Build history of the part. All positions in model axes, mm. Face numbers are marked on the shaded views. A direction names the side the tool comes from. Give positions to 0.01 mm unless a question says otherwise; leave off trailing zeros. Loops run counter-clockwise (first coordinate to the right, second up) from the corner with the lowest first, then second, coordinate; pieces in that order, holes last. Notation, with made-up numbers: (61.25, -15.75) -> (96.25, -15.75) arc R14 ccw to (96.25, -9.75) -> close; hole circle Ø10 at (57, 53.25). An arc over 180 degrees is marked (long way). Answer as a JSON object with one key per item and string values. Group by question number.
Q1. Band-saw the part on D-D, the plane x = 16.5. Write the cut outline in (y, z), plus the area to 3 significant figures.
Q2. Drop flat-ended pins along their axis: pin 1 (2 mm diameter, centred on x = -13, z = -2, fed in from +Y); pin 2 (2 mm diameter, centred on x = -8.5, y = 1, fed in from -Z); pin 3 (2 mm diameter, centred on y = 2.5, z = -8, fed in from -X); pin 4 (1.8 mm diameter, centred on y = 2.5, z = 5, fed in from -X). Give the stop position or say it passes through.
Q3. Wall check: probe 1 along X at (y, z) = (1.75, -5); probe 2 along X at (y, z) = (3.7, 5.5); probe 3 along Z at (x, y) = (13.5, 2.7). Give the ranges that are in metal, low to high. Write a range as from..to.
Q4. Band-saw the part on B-B, the plane y = 3. Write the cut outline in (x, z), plus the area to 3 significant figures.
Q5. Two-plate mould, pull along Z, no slides. Class the marked faces 4, 5, 6 and 7: pulls with the +Z half, pulls with the -Z half, needs draft (parallel to the pull), parting line crosses it, or undercut.
Q6. Band-saw the part on A-A, the plane x = 0. Write the cut outline in (y, z).
Q7. Band-saw the part on C-C, the plane x = -16. Write the cut outline in (y, z), plus the area to 3 significant figures.
Q8. Tool access for the marked faces 1, 2 and 3: list every direction of +Z, -Z, +X, -X, +Y, -Y with a clear straight run to the whole face (end or side of a thin tool).
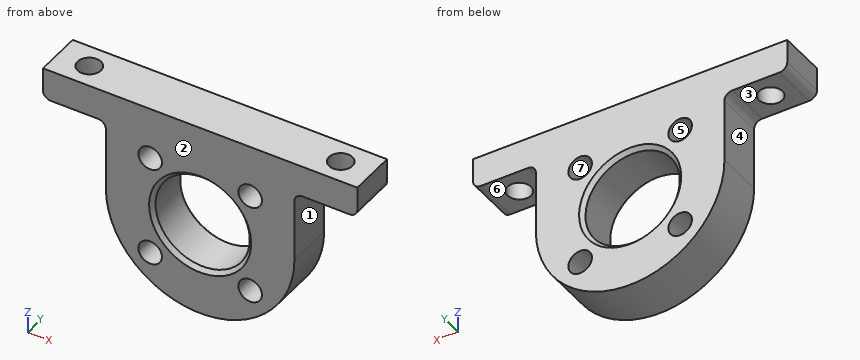
from build123d import *

# Parameters (mm, degrees)
EXTRUDE_1_DEPTH     = 6
SKETCH_2_R          = 6
CUT_EXTRUDE_1_DEPTH = 6
SKETCH_3_R          = 1.5
CUT_EXTRUDE_2_DEPTH = 6
SKETCH_9_W          = 40
SKETCH_9_H          = 6
EXTRUDE_4_DEPTH     = 4
SKETCH_10_R         = 1.5
CUT_EXTRUDE_4_DEPTH = 5
FILLET_2_R          = 1
CHAMFER_1_SIZE      = 0.5


with BuildPart() as part:
    # 草图1 → 凸台-拉伸1 (new body)
    with BuildSketch(Plane(origin=(0, 0, 0), x_dir=(1, 0, 0), z_dir=(0, 1, 0))):
        with BuildLine():
            Line((-12, 0), (-12, -13))
            Line((-12, -13), (12, -13))
            Line((12, -13), (12, 0))
            ThreePointArc((12, 0), (0, 12), (-12, 0))
        make_face()
    extrude(amount=EXTRUDE_1_DEPTH)

    # 草图2 → 切除-拉伸1 (cut)
    with BuildSketch(Plane(origin=(0, 6, 0), x_dir=(1, 0, 0), z_dir=(0, 1, 0))):
        with Locations(Location((0, 0, 0), (0, 0, 270))):
            Circle(SKETCH_2_R)
    extrude(amount=-CUT_EXTRUDE_1_DEPTH, mode=Mode.SUBTRACT)

    # 草图3 → 切除-拉伸2 (cut)
    with BuildSketch(Plane(origin=(0, 6, 0), x_dir=(1, 0, 0), z_dir=(0, 1, 0))):
        with Locations(Location((-6.363961031, 6.363961031, 0), (0, 0, 270))):
            Circle(SKETCH_3_R)
        with Locations(Location((6.363961031, 6.363961031, 0), (0, 0, 270))):
            Circle(SKETCH_3_R)
        with Locations(Location((6.363961031, -6.363961031, 0), (0, 0, 270))):
            Circle(SKETCH_3_R)
        with Locations(Location((-6.363961031, -6.363961031, 0), (0, 0, 270))):
            Circle(SKETCH_3_R)
    extrude(amount=-CUT_EXTRUDE_2_DEPTH, mode=Mode.SUBTRACT)

    # 草图9 → 凸台-拉伸4 (add)
    with BuildSketch(Plane.XY.offset(13)):
        with Locations((0, 3)):
            Rectangle(SKETCH_9_W, SKETCH_9_H)
    extrude(amount=-EXTRUDE_4_DEPTH)

    # 草图10 → 切除-拉伸4 (cut)
    with BuildSketch(Plane.XY.offset(13)):
        with Locations((-16, 3)):
            Circle(SKETCH_10_R)
        with Locations((16, 3)):
            Circle(SKETCH_10_R)
    extrude(amount=-CUT_EXTRUDE_4_DEPTH, mode=Mode.SUBTRACT)

    # 圆角2
    fillet_2_edges = [part.edges().sort_by_distance(p)[0] for p in [
        (-12, 3, 9),
        (12, 3, 9),
        (-20, 3, 9),
        (20, 3, 9),
    ]]
    fillet(fillet_2_edges, radius=FILLET_2_R)

    # 倒角1
    chamfer_1_edges = [part.edges().sort_by_distance(p)[0] for p in [
        (0, 0, -6),
        (0, 6, -6),
    ]]
    chamfer(chamfer_1_edges, length=CHAMFER_1_SIZE)


solid = part.part
Worked answers:
{
 "1": {"outline": "(0, 9) -> (1.59, 9) -> (1.59, 13) -> (0, 13) -> close; (4.41, 9) -> (6, 9) -> (6, 13) -> (4.41, 13) -> close", "area": "12.7 mm2"},
 "2": {"pin 1": "through", "pin 2": "z = -9.37", "pin 3": "x = -9.75", "pin 4": "x = -12"},
 "3": {"probe 1": "-10.91..-6.99, -5.74..-3.32, 3.32..5.74, 6.99..10.91", "probe 2": "-12..-7.59, -5.14..-2.4, 2.4..5.14, 7.59..12", "probe 3": "9..13"},
 "4": {"outline": "(-20, 10) arc R1 ccw to (-19, 9) -> (-17.5, 9) -> (-17.5, 13) -> (-20, 13) -> close; (-14.5, 9) -> (-13, 9) arc R1 cw to (-12, 8) -> (-12, 0) arc R12 ccw to (12, 0) -> (12, 8) arc R1 cw to (13, 9) -> (14.5, 9) -> (14.5, 13) -> (-14.5, 13) -> close; (17.5, 9) -> (19, 9) arc R1 ccw to (20, 10) -> (20, 13) -> (17.5, 13) -> close; hole circle Ø3 at (-6.36, -6.36); hole circle Ø3 at (-6.36, 6.36); hole circle Ø12 at (0, 0); hole circle Ø3 at (6.36, -6.36); hole circle Ø3 at (6.36, 6.36)", "area": "437 mm2"},
 "5": {"face 4": "needs draft", "face 5": "undercut", "face 6": "pulls with the -Z half", "face 7": "undercut"},
 "6": {"outline": "(0, -12) -> (6, -12) -> (6, -6.5) -> (5.5, -6) -> (0.5, -6) -> (0, -6.5) -> close; (0, 6.5) -> (0.5, 6) -> (5.5, 6) -> (6, 6.5) -> (6, 13) -> (0, 13) -> close"},
 "7": {"outline": "(0, 9) -> (1.5, 9) -> (1.5, 13) -> (0, 13) -> close; (4.5, 9) -> (6, 9) -> (6, 13) -> (4.5, 13) -> close", "area": "12.0 mm2"},
 "8": {"face 1": "-Z, +X, +Y, -Y", "face 2": "+Z, -Z, +X, -X, -Y", "face 3": "-Z, -X, +Y, -Y"}
}
